The model under review builds one solid part; all positions refer to its coordinate system, in mm. Face numbers are marked on the shaded views. Give positions to 0.01 mm unless a question says otherwise; leave off trailing zeros. Order: outer loops, then holes, each group sorted by start corner. A loop starts at its lowest first (then second) coordinate and runs counter-clockwise, first axis right, second up. Notation, with made-up numbers: (-23, 53.25) -> (-14, 53.25) arc R16 ccw to (-14, 73.25) -> close; hole circle Ø10 at (-8, 33). An arc over 180 degrees is marked (long way). Use one line per item in the form item = value.
```python
from build123d import *

# Parameters (mm, degrees)
SKETCH_1_R          = 37.5
EXTRUDE_1_DEPTH     = 2
SKETCH_2_R          = 1.75
CUT_EXTRUDE_1_DEPTH = 2
SKETCH_3_R          = 16.5
EXTRUDE_2_DEPTH     = 5
SKETCH_4_R          = 9.75
SKETCH_4_R_2        = 1.8
CUT_EXTRUDE_2_DEPTH = 7


with BuildPart() as part:
    # Эскиз1 → Бобышка-Вытянуть1 (new body)
    with BuildSketch(Plane.XY):
        Circle(SKETCH_1_R)
    extrude(amount=EXTRUDE_1_DEPTH)

    # Эскиз2 → Вырез-Вытянуть1 (cut)
    with BuildSketch(Plane.XY.offset(2)):
        with Locations((0, 32.5)):
            Circle(SKETCH_2_R)
        with Locations((32.5, 0)):
            Circle(SKETCH_2_R)
        with Locations((0, -32.5)):
            Circle(SKETCH_2_R)
        with Locations((-32.5, 0)):
            Circle(SKETCH_2_R)
    extrude(amount=-CUT_EXTRUDE_1_DEPTH, mode=Mode.SUBTRACT)

    # Эскиз3 → Бобышка-Вытянуть2 (add)
    with BuildSketch(Plane.XY.offset(2)):
        Circle(SKETCH_3_R)
    extrude(amount=EXTRUDE_2_DEPTH)

    # Эскиз4 → Вырез-Вытянуть2 (cut)
    with BuildSketch(Plane.XY.offset(7)):
        Circle(SKETCH_4_R)
        with Locations((0, 12.6)):
            Circle(SKETCH_4_R_2)
        with Locations((10.911920088, -6.3)):
            Circle(SKETCH_4_R_2)
        with Locations((-10.911920088, -6.3)):
            Circle(SKETCH_4_R_2)
    extrude(amount=-CUT_EXTRUDE_2_DEPTH, mode=Mode.SUBTRACT)


solid = part.part
```
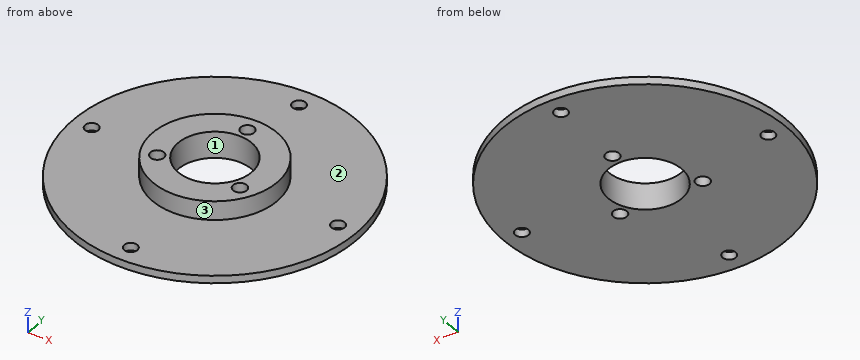
1. Add section B-B on z = 5.75. Give the boundary of the cut face in (x, y).
Values:
outline = circle Ø33 at (0, 0); hole circle Ø3.6 at (-10.91, -6.3); hole circle Ø19.5 at (0, 0); hole circle Ø3.6 at (0, 12.6); hole circle Ø3.6 at (10.91, -6.3)
2. Add section D-D on y = 12.6. Give the boundary of the cut face in (x, z), then the cut area to 3 significant figures.
Values:
outline = (-35.32, 0) -> (-1.8, 0) -> (-1.8, 7) -> (-10.65, 7) -> (-10.65, 2) -> (-35.32, 2) -> close; (1.8, 0) -> (35.32, 0) -> (35.32, 2) -> (10.65, 2) -> (10.65, 7) -> (1.8, 7) -> close
area = 223 mm^2
3. For L1, parallel to Y at x = 0, z = 0.8; L2, parallel to Z at x = 18, y = 32; L3, parallel to Y at x = -31, z = 1.75, list the stretches that pass through material, from the lowest coordinate up.
Values:
L1 = -37.5 to -34.25, -30.75 to -9.75, 9.75 to 10.8, 14.4 to 30.75, 34.25 to 37.5
L2 = 0 to 2
L3 = -21.1 to -0.9, 0.9 to 21.1
4. Add section C-C on x = 3.5. Give the boundary of the cut face in (y, z), then the cut area to 3 significant figures.
Values:
outline = (-37.34, 0) -> (-9.1, 0) -> (-9.1, 7) -> (-16.12, 7) -> (-16.12, 2) -> (-37.34, 2) -> close; (9.1, 0) -> (37.34, 0) -> (37.34, 2) -> (16.12, 2) -> (16.12, 7) -> (9.1, 7) -> close
area = 183 mm^2
5. The part is to be moulded in two halves that separate along X. For the marked faces 1, 2 and 3, say which applies: +X half, -X half, draft (parallel to the pull), parting line (faces both ways), or undercut.
Values:
face_1 = undercut
face_2 = draft
face_3 = parting line
6. For pin 1 Ø3 at (y, z) = (-19.5, 6.5) entering from -X; pin 2 Ø4 at (x, y) = (0, -32.5) entering from +Z; pin 3 Ø2 at (y, z) = (-12.5, 4) entering from -X; pin 4 Ø2 at (y, z) = (8, 4.5) entering from -X, all flat-tipped, find the tip position at first contact; note any pin that passes through.
Values:
pin_1 = through
pin_2 = 2
pin_3 = -11.83
pin_4 = -14.94
7. Add section A-A on y = 0. Give the boundary of the cut face in (x, z), then the cut area to 4 significant figures.
Values:
outline = (-37.5, 0) -> (-34.25, 0) -> (-34.25, 2) -> (-37.5, 2) -> close; (-30.75, 0) -> (-9.75, 0) -> (-9.75, 7) -> (-16.5, 7) -> (-16.5, 2) -> (-30.75, 2) -> close; (9.75, 0) -> (30.75, 0) -> (30.75, 2) -> (16.5, 2) -> (16.5, 7) -> (9.75, 7) -> close; (34.25, 0) -> (37.5, 0) -> (37.5, 2) -> (34.25, 2) -> close
area = 164.5 mm^2
